```python
from build123d import *

# Parameters (mm, degrees)
F0_W     = 50
F0_H     = 100
F0_H_2   = 1
F1_DEPTH = 40
F2_DEPTH = 3
F3_DEPTH = 2


with BuildPart() as f1:
    # F0 (on Top) → F1 (new body)
    with BuildSketch(Plane.XY):
        Polygon((-25, -50), (-25, 50), (-25, 51), (-27, 51), (-27, -52), (131, -52), (131, 51), (25, 51), (25, 50), (25, -50), align=None)
        with Locations((52, 0)):
            Rectangle(F0_W, F0_H, mode=Mode.SUBTRACT)
        with Locations((104, 0)):
            Rectangle(F0_W, F0_H, mode=Mode.SUBTRACT)
        with Locations((0, 50.5)):
            Rectangle(F0_W, F0_H_2)
    extrude(amount=F1_DEPTH)

    # F0 (on Top) → F2 (join)
    with BuildSketch(Plane.XY):
        Rectangle(F0_W, F0_H)
        Polygon((-20, -45), (-20, 34.40983), (19.704915, -45), align=None, mode=Mode.SUBTRACT)
        Polygon((20, -34.40983), (-19.704915, 45), (20, 45), align=None, mode=Mode.SUBTRACT)
        with Locations((52, 0)):
            Rectangle(F0_W, F0_H)
        Polygon((32, 34.40983), (71.704915, -45), (32, -45), align=None, mode=Mode.SUBTRACT)
        Polygon((72, -34.40983), (32.295085, 45), (72, 45), align=None, mode=Mode.SUBTRACT)
        with Locations((104, 0)):
            Rectangle(F0_W, F0_H)
        Polygon((84, 34.40983), (123.704915, -45), (84, -45), align=None, mode=Mode.SUBTRACT)
        Polygon((124, -34.40983), (84.295085, 45), (124, 45), align=None, mode=Mode.SUBTRACT)
    extrude(amount=F2_DEPTH)

    # F0 (on Top) → F3 (join)
    with BuildSketch(Plane.XY):
        Polygon((20, 45), (-19.704915, 45), (20, -34.40983), align=None)
        Polygon((19.704915, -45), (-20, 34.40983), (-20, -45), align=None)
        Polygon((32, -45), (71.704915, -45), (32, 34.40983), align=None)
        Polygon((72, 45), (32.295085, 45), (72, -34.40983), align=None)
        Polygon((124, 45), (84.295085, 45), (124, -34.40983), align=None)
        Polygon((84, -45), (123.704915, -45), (84, 34.40983), align=None)
    extrude(amount=F3_DEPTH)


solid = f1.part
```
Input: part model. Units: mm. Frame: model coordinates. A direction names the side the tool comes from. Coordinates: 2 decimals unless noted, no trailing zeros. Loops run counter-clockwise (first coordinate to the right, second up) from the corner with the lowest first, then second, coordinate; pieces in that order, holes last.
Q1. Contact query for flat-ended pins moving along their axis: pin 1 (6 mm diameter, centred on x = 86.5, y = 27.5, fed in from +Z); pin 2 (1 mm diameter, centred on x = 87.5, y = -12.5, fed in from +Z). Output: stop coordinate, or through.
Results are:
pin 1: stops at z = 3
pin 2: stops at z = 2
Q2. Section B-B, the plane x = 30. Return the cut outline in (y, z).
Results are:
outline: (-52, 0) - (51, 0) - (51, 40) - (50, 40) - (50, 3) - (-50, 3) - (-50, 40) - (-52, 40) - close
Q3. Section A-A, the plane z = 11. Return the cut outline in (x, y), and give its area (3 significant figures).
Results are:
outline: (-27, -52) - (131, -52) - (131, 51) - (-27, 51) - close; hole (-25, -50) - (25, -50) - (25, 50) - (-25, 50) - close; hole (27, -50) - (77, -50) - (77, 50) - (27, 50) - close; hole (79, -50) - (129, -50) - (129, 50) - (79, 50) - close
area: 1,270 mm2
Q4. Section C-C, the plane y = -36.5. Return the cut outline in (x, z), and give its area (3 significant figures).
Results are:
outline: (-27, 0) - (131, 0) - (131, 40) - (129, 40) - (129, 3) - (119.45, 3) - (119.45, 2) - (84, 2) - (84, 3) - (79, 3) - (79, 40) - (77, 40) - (77, 3) - (67.45, 3) - (67.45, 2) - (32, 2) - (32, 3) - (27, 3) - (27, 40) - (25, 40) - (25, 3) - (15.45, 3) - (15.45, 2) - (-20, 2) - (-20, 3) - (-25, 3) - (-25, 40) - (-27, 40) - close
area: 664 mm2
Q5. Mould query, pull axis Y, two halves, no side actions, for faces 3 (the flat face through (51, 0, 0)), 4 (the flat face through (53, 51, 20)), 5 (the flat face through (-9, -22, 2)). Classes: +Y half, -Y half, draft (parallel to the pull), parting line (faces both ways), or undercut.
Results are:
face 3: draft
face 4: +Y half
face 5: undercut
Q6. Line query: line 1 along X through (y, z) = (8.5, 22); line 2 along Y through (x, z) = (-17.5, 34); line 3 along Z through (x, y) = (31, 0.5). Output: solid intervals per line, ascending.
Results are:
line 1: x = -27 to -25, 25 to 27, 77 to 79, 129 to 131
line 2: y = -52 to -50, 50 to 51
line 3: z = 0 to 3
Q7. Section D-D, the plane x = 58.5. Return the cut outline in (y, z), and give its area (3 significant figures).
Results are:
outline: (-52, 0) - (51, 0) - (51, 40) - (50, 40) - (50, 3) - (45, 3) - (45, 2) - (-7.41, 2) - (-7.41, 3) - (-18.59, 3) - (-18.59, 2) - (-45, 2) - (-45, 3) - (-50, 3) - (-50, 40) - (-52, 40) - close
area: 341 mm2
Q8. Set-up query: faces 1 (the flat face through (95, -22, 2)), 2 (the flat face through (-27, 0, 20)). Return all of +Z, -Z, +X, -X, +Y, -Y with unobstructed straight access to the full face (end or side cutting, diameter ignored); none if empty.
Results are:
face 1: +Z
face 2: +Z, -Z, -X, +Y, -Y
